from build123d import *

# Parameters (mm, degrees)
SKETCH1_W           = 20
SKETCH1_H           = 30
SKETCH1_R           = 3.25
BOSS_EXTRUDE1_DEPTH = 3
SKETCH2_W           = 20
SKETCH2_H           = 3
BOSS_EXTRUDE2_DEPTH = 27
SKETCH3_R           = 3.25
CUT_EXTRUDE1_DEPTH  = 46.044422518
BOSS_EXTRUDE3_DEPTH = 3
FILLET1_R           = 1


with BuildPart() as part:
    # Sketch1 → Boss-Extrude1 (new body)
    with BuildSketch(Plane(origin=(0, 0, 0), x_dir=(1, 0, 0), z_dir=(0, 1, 0))):
        with Locations((-10, 15)):
            Rectangle(SKETCH1_W, SKETCH1_H)
        with Locations(Location((-10, 10, 0), (0, 0, 270))):
            Circle(SKETCH1_R, mode=Mode.SUBTRACT)
    extrude(amount=BOSS_EXTRUDE1_DEPTH)

    # Sketch2 → Boss-Extrude2 (add)
    with BuildSketch(Plane(origin=(0, 3, 0), x_dir=(1, 0, 0), z_dir=(0, 1, 0))):
        with Locations((-10, 28.5)):
            Rectangle(SKETCH2_W, SKETCH2_H)
    extrude(amount=BOSS_EXTRUDE2_DEPTH)

    # Sketch3 → Cut-Extrude1 (cut, through all)
    with BuildSketch(Plane.XY.offset(-27)):
        with Locations((-10, 20)):
            Circle(SKETCH3_R)
    extrude(amount=-CUT_EXTRUDE1_DEPTH, mode=Mode.SUBTRACT)

    # Sketch5 → Boss-Extrude3 (add)
    with BuildSketch(Plane(origin=(0, 0, 0), x_dir=(0, 0, -1), z_dir=(1, 0, 0))):
        Polygon((12, 3), (27, 18), (27, 3), align=None)
    boss_extrude3 = extrude(amount=-BOSS_EXTRUDE3_DEPTH)

    # Mirror1: Boss-Extrude3 across plane
    add(boss_extrude3.mirror(Plane.ZY.offset(10)))

    # Fillet1
    fillet1_edges = [part.edges().sort_by_distance(p)[0] for p in [
        (-10, 3, 0),
        (-20, 24, -27),
        (0, 24, -27),
        (-20, 30, -28.5),
        (-10, 30, -27),
        (0, 30, -28.5),
        (-10, 30, -30),
        (0, 10.5, -19.5),
        (-20, 3, -6),
        (-20, 10.5, -19.5),
        (0, 3, -6),
        (-10, 0, 0),
        (-20, 0, -15),
        (-10, 0, -30),
        (0, 0, -15),
        (0, 1.5, 0),
        (-20, 1.5, 0),
        (-20, 15, -30),
        (0, 15, -30),
    ]]
    fillet(fillet1_edges, radius=FILLET1_R)


solid = part.part
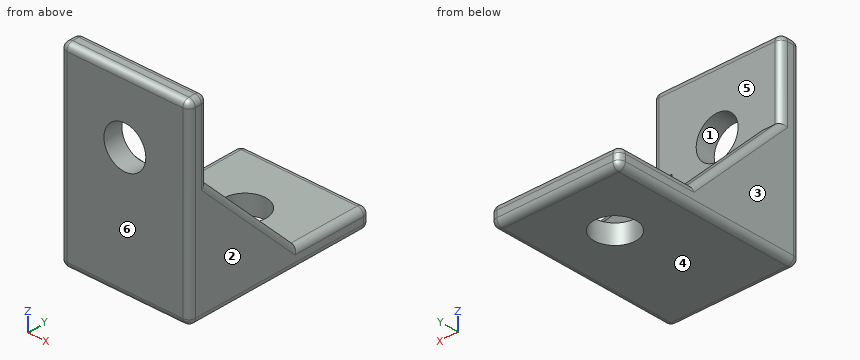
The model under review builds one solid part; all positions refer to its coordinate system, in mm. Face numbers are marked on the shaded views. A direction names the side the tool comes from. Coordinates: 2 decimals unless noted, no trailing zeros. Order: outer loops, then holes, each group sorted by start corner. A loop starts at its lowest first (then second) coordinate and runs counter-clockwise, first axis right, second up. Notation, with made-up numbers: (-26.75, 11.5) -> (31.25, 11.5) arc R13 ccw to (31.25, 35.5) -> close; hole circle Ø4 at (51.5, -26.5). An arc over 180 degrees is marked (long way). Answer in a Markdown table with one row per item.
(1) Consider section C-C (z = -11). Write out the cut boundary in (x, y), plus the area to 3 significant figures.
Answers:
| item | result |
|---|---|
| outline | (-20, 1) arc R1 ccw to (-19, 0) -> (-13.09, 0) -> (-13.09, 3) -> (-19, 3) arc R1 ccw to (-20, 2) -> close; (-6.91, 0) -> (-1, 0) arc R1 ccw to (0, 1) -> (0, 2) arc R1 ccw to (-1, 3) -> (-6.91, 3) -> close |
| area | 40.6 mm² |
(2) Consider section A-A (y = 20). Write out the cut boundary in (x, z), plus the area to 3 significant figures.
Answers:
| item | result |
|---|---|
| outline | (-20, -29) arc R1 ccw to (-19, -30) -> (-13.25, -30) -> (-13.25, -27) -> (-19, -27) arc R1 ccw to (-20, -28) -> close; (-6.75, -30) -> (-1, -30) arc R1 ccw to (0, -29) -> (0, -28) arc R1 ccw to (-1, -27) -> (-6.75, -27) -> close |
| area | 39.6 mm² |
(3) Consider section D-D (x = -17.5). Write out the cut boundary in (y, z), plus the area to 3 significant figures.
Answers:
| item | result |
|---|---|
| outline | (0, -29) arc R1 ccw to (1, -30) -> (29, -30) arc R1 ccw to (30, -29) -> (30, -28) arc R1 ccw to (29, -27) -> (18, -27) -> (3, -12) -> (3, -1) arc R1 ccw to (2, 0) -> (1, 0) arc R1 ccw to (0, -1) -> close |
| area | 282 mm² |
(4) Wall thickness on line 1 along X through (y, z) = (1.1, -10); line 2 along X through (y, z) = (6.5, -23.25); line 3 along Y through (x, z) = (-3.5, -12): over which ranges is each line inside the solid? List them lowest first.
Answers:
| item | result |
|---|---|
| line 1 | -20 to -13.25, -6.75 to 0 |
| line 2 | -20 to -17, -3 to 0 |
| line 3 | 0 to 3 |
(5) Insertion check: pin 1 (8.5 mm diameter, centred on x = -10, y = 20, fed in from +Z); pin 2 (10 mm diameter, centred on y = 5.5, z = -11, fed in from -X); pin 3 (5 mm diameter, centred on x = -10, z = -10, fed in from +Y) (3 decimals); pin 4 (5.5 mm diameter, centred on x = -9, z = -16.5, fed in from +Y). Each pin has a flat end and moves straight along its axis. Give the tip position at first contact, or say it passes through.
Answers:
| item | result |
|---|---|
| pin 1 | z = -27 |
| pin 2 | x = -20 |
| pin 3 | through |
| pin 4 | y = 3 |
(6) Consider section B-B (x = -7.25). Write out the cut boundary in (y, z), plus the area to 3 significant figures.
Answers:
| item | result |
|---|---|
| outline | (0, -29) arc R1 ccw to (1, -30) -> (18.27, -30) -> (18.27, -27) -> (3, -27) -> (3, -11.73) -> (0, -11.73) -> close; (0, -8.27) -> (3, -8.27) -> (3, -1) arc R1 ccw to (2, 0) -> (1, 0) arc R1 ccw to (0, -1) -> close; (21.73, -30) -> (29, -30) arc R1 ccw to (30, -29) -> (30, -28) arc R1 ccw to (29, -27) -> (21.73, -27) -> close |
| area | 149 mm² |
(7) Machinability: for the marked faces 5 and 6, which of the approach directions +Z, -Z, +X, -X, +Y, -Y give a long, thin tool a straight path to every point of the face, cutting with its end or side? Answer none if there is none.
Answers:
| item | result |
|---|---|
| face 5 | +Z, +Y |
| face 6 | +Z, -Z, +X, -X, -Y |
(8) The part is to be moulded in two halves that separate along X. For the marked faces 1, 2, 3 and 4, say which applies: +X half, -X half, draft (parallel to the pull), parting line (faces both ways), or undercut.
Answers:
| item | result |
|---|---|
| face 1 | undercut |
| face 2 | +X half |
| face 3 | -X half |
| face 4 | draft |
